Autodesk Inventor part; units mm, degrees
ref_plane "YZ Plane" through (0, 0, 0) normal (1, 0, 0) x (0, 1, 0)
ref_plane "XZ Plane" through (0, 0, 0) normal (0, 1, 0) x (-1, 0, 0)
ref_plane "XY Plane" through (0, 0, 0) normal (0, 0, 1) x (1, 0, 0)
sketch "Sketch1" plane through (0, 0, 0) normal (0, 1, 0) x (-1, 0, 0)
  circle A0 centre (0, 0) radius 63.465
  circle A1 centre (0, 0) radius 55.575
  dimension "d0" = 126.93
  dimension "d1" = 111.15
extrude "Extrusion1" add sketch "Sketch1" along normal blind 55.37
sketch "Sketch2" plane through (0, 55.37, 0) normal (0, 1, 0) x (1, 0, 0)
  circle A0 centre (0, 0) radius 63.465
  circle A1 centre (0, 0) radius 45.115
  dimension "d4" = 90.23
extrude "Extrusion2" add sketch "Sketch2" against normal blind 5
fillet "Fillet1" radius 5 1 edges at (63.465, 55.37, 0)
sketch "Sketch3" plane through (0, 0, 0) normal (0, -1, 0) x (1, 0, 0)
  circle A0 centre (0, 0) radius 63.465
  circle A1 centre (63.465, 0) radius 4.5231
extrude "Extrusion3" add sketch "Sketch3" against normal blind 37.92 contours A0 A1 | A0 A1 picked at (62.045, -1.0257) picked at (64.8107, -1.1706)
pattern_circular "Circular Pattern1" count 12 over 360 about axis through (0, 0, 0) along (0, 1, 0) of "Extrusion3"
properties part number "00_Compression_Coupling_3inch_KingBrothers_CPC-3000_locking"
CAD build for the part. Positions are in the model's coordinates, mm. A direction names the side the tool comes from. Coordinates: 2 decimals unless noted, no trailing zeros. Write each loop counter-clockwise with the first axis right and the second up, starting at its lowest first coordinate (ties: lowest second). Pieces come first, ordered by that corner, then holes. Notation, with made-up numbers: (57.5, 38.5) - (113.5, 38.5) arc R29 cw to (113.5, 58.5) - close; hole circle Ø1 at (59, 78). An arc over 180 degrees is marked (long way). Use a Markdown table: item, result. Add a question column.
Item 1: Band-saw the part on B-B, the plane z = 0. Give the cut face in (x, y) (3 decimals).
Item 2: 3-axis set-ups, long thin cutter, end or side, ignore diameter. For faces 1 (the face through (56, 37.92, 33)), 2 (the face through (-56, 37.92, 32)), 3 (the face through (-56, 37.92, -33)), 4 (the face through (0, 50.37, -46)): which of +Z, -Z, +X, -X, +Y, -Y reach the whole face in a straight line?
Item 3: Mould opens along Z. For faces 5 (the face through (0, 37.92, 65)), 6 (the face through (-58.83, 18.69, 34.08)) say: pulls with the +Z half, pulls with the -Z half, needs draft (parallel to the pull), parting line crosses it, or undercut.
Item 4: Band-saw the part on A-A, the plane x = 0. Give the cut face in (y, z) (3 decimals), and give its area (3 significant figures).
Item 5: Drill centre lines: L1, parallel to X at y = 40, z = 0 (3 decimals); L2, parallel to X at y = 5.5, z = 17.5; L3, parallel to Z at x = 0, y = 53 (3 decimals). Where is each one in solid material? Low to high. Write a range as from..to.
Item 6: Flat gauge pins, fed straight in: pin 1 (3 mm diameter, centred on x = -32, y = 35, fed in from +Z); pin 2 (12 mm diameter, centred on y = 17, z = 21.5, fed in from -X); pin 3 (5.5 mm diameter, centred on x = -34, z = 55.5, fed in from +Y). Where does each tip first touch, or does it go through?
Numbers:
| question | item | result |
|---|---|---|
| 1 | outline | (-67.988, 0) - (-55.575, 0) - (-55.575, 50.37) - (-45.115, 50.37) - (-45.115, 55.37) - (-58.465, 55.37) arc R5 ccw to (-63.465, 50.37) - (-63.465, 37.92) - (-67.988, 37.92) - close; (45.115, 50.37) - (55.575, 50.37) - (55.575, 0) - (67.988, 0) - (67.988, 37.92) - (63.465, 37.92) - (63.465, 50.37) arc R5 ccw to (58.465, 55.37) - (45.115, 55.37) - close |
| 2 | face 1 | +Z, +X, +Y |
| 2 | face 2 | +Z, -X, +Y |
| 2 | face 3 | -Z, -X, +Y |
| 2 | face 4 | -Y |
| 3 | face 5 | needs draft |
| 3 | face 6 | undercut |
| 4 | outline | (0, -67.988) - (37.92, -67.988) - (37.92, -63.465) - (50.37, -63.465) arc R5 ccw to (55.37, -58.465) - (55.37, -45.115) - (50.37, -45.115) - (50.37, -55.575) - (0, -55.575) - close; (0, 55.575) - (50.37, 55.575) - (50.37, 45.115) - (55.37, 45.115) - (55.37, 58.465) arc R5 ccw to (50.37, 63.465) - (37.92, 63.465) - (37.92, 67.988) - (0, 67.988) - close |
| 4 | area | 1,310 mm2 |
| 5 | L1 | -63.465..-55.575, 55.575..63.465 |
| 5 | L2 | -61..-52.75, 52.75..61 |
| 5 | L3 | -62.717..-45.115, 45.115..62.717 |
| 6 | pin 1 | z = 59.49 |
| 6 | pin 2 | x = -61.54 |
| 6 | pin 3 | y = 53.53 |
